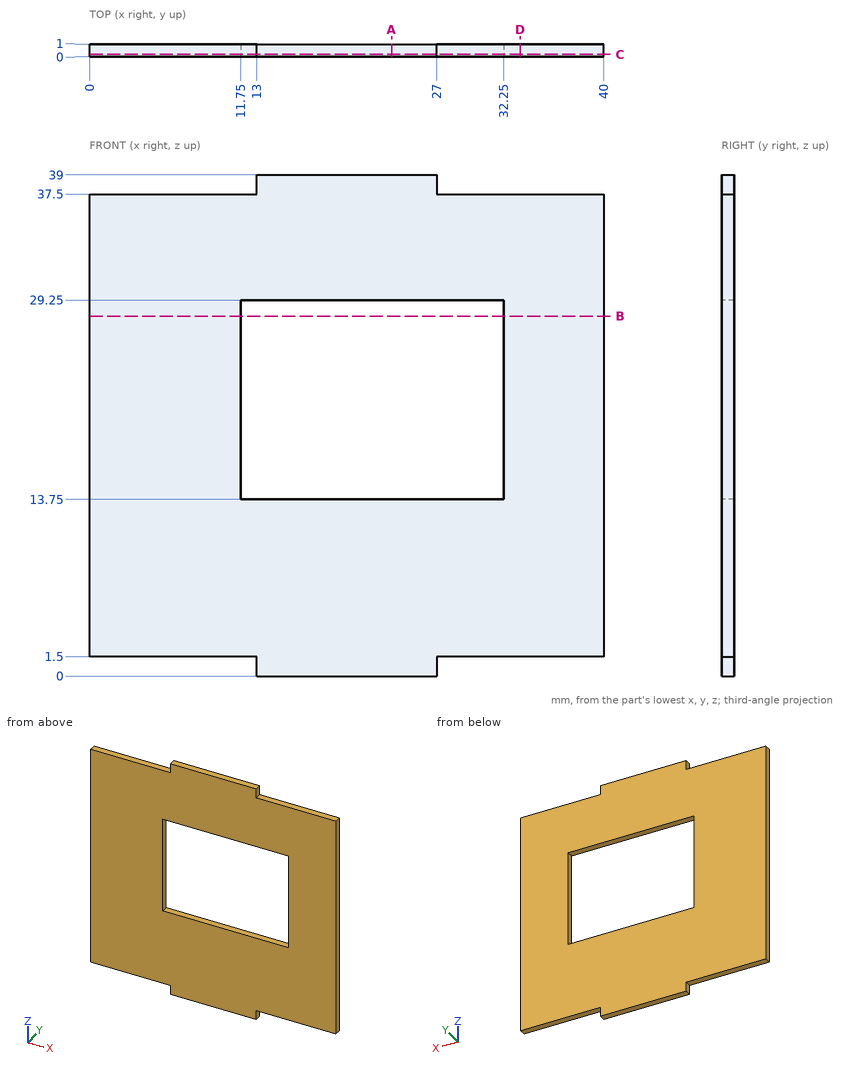
Input: dimensioned drawing with shaded views. Units: mm. Origin: part minimum x, y, z. Coordinates: 2 decimals unless noted, no trailing zeros. Loops run counter-clockwise (first coordinate to the right, second up) from the corner with the lowest first, then second, coordinate; pieces in that order, holes last. Notation, with made-up numbers: (-32.5, -31.5) -> (25.5, -31.5) arc R19 ccw to (25.5, 4.5) -> close; hole circle Ø2 at (48.5, 34.25). An arc over 180 degrees is marked (long way). Use a Markdown table: item, result. Add a question column.
(1) Section query D-D, the plane x = 33.5. Return loops of the section in (y, z).
(2) Section query B-B, the plane z = 28. Return loops of the section in (x, y).
(3) Section query A-A, the plane x = 23.5. Return loops of the section in (y, z), plus the area to 3 significant figures.
(4) Section query C-C, the plane y = 0.2. Return loops of the section in (x, z).
(5) Line query: line 1 along X through (y, z) = (0.3, 27); line 2 along Z through (x, y) = (31, 0.8); line 3 along Z through (x, y) = (18, 0.1). Output: solid intervals per line, ascending.
(6) Pin query (flat end, axial travel): pin 1 Ø0.5 at (x, y) = (7.5, 0.5) entering from +Z; pin 2 Ø0.5 at (y, z) = (0.5, 1) entering from +X. Return the tip coordinate at first contact, or that it passes through.
Answer:
| question | item | result |
|---|---|---|
| 1 | outline | (0, 1.5) -> (1, 1.5) -> (1, 37.5) -> (0, 37.5) -> close |
| 2 | outline | (0, 0) -> (11.75, 0) -> (11.75, 1) -> (0, 1) -> close; (32.25, 0) -> (40, 0) -> (40, 1) -> (32.25, 1) -> close |
| 3 | outline | (0, 0) -> (1, 0) -> (1, 13.75) -> (0, 13.75) -> close; (0, 29.25) -> (1, 29.25) -> (1, 39) -> (0, 39) -> close |
| 3 | area | 23.5 mm^2 |
| 4 | outline | (0, 1.5) -> (13, 1.5) -> (13, 0) -> (27, 0) -> (27, 1.5) -> (40, 1.5) -> (40, 37.5) -> (27, 37.5) -> (27, 39) -> (13, 39) -> (13, 37.5) -> (0, 37.5) -> close; hole (11.75, 13.75) -> (32.25, 13.75) -> (32.25, 29.25) -> (11.75, 29.25) -> close |
| 5 | line 1 | x = 0 to 11.75, 32.25 to 40 |
| 5 | line 2 | z = 1.5 to 13.75, 29.25 to 37.5 |
| 5 | line 3 | z = 0 to 13.75, 29.25 to 39 |
| 6 | pin 1 | stops at z = 37.5 |
| 6 | pin 2 | stops at x = 27 |
